Design review of the part built by this model. Coordinates are the model's own, in mm. Face numbers are marked on the shaded views. A direction names the side the tool comes from. Give positions to 0.01 mm unless a question says otherwise; leave off trailing zeros. Order: outer loops, then holes, each group sorted by start corner. A loop starts at its lowest first (then second) coordinate and runs counter-clockwise, first axis right, second up.
```python
from build123d import *

# Parameters (mm, degrees)
F0_W     = 149.768152
F0_H     = 37.856524
F1_DEPTH = 17
F2_W     = 12.044117
F2_H     = 10.517036
F3_DEPTH = 68.7
F2_W_2   = 49.102947
F2_H_2   = 8.573649
F4_DEPTH = 6.2


with BuildPart() as f1:
    # F0 (on Top) → F1 (new body)
    with BuildSketch(Plane.XY):
        with Locations((-0.134293, 0.313039)):
            Rectangle(F0_W, F0_H)
    extrude(amount=F1_DEPTH)

    # F2 (on face) → F3 (join)
    with BuildSketch(Plane.XY.offset(17)):
        with Locations((-0.08639, 13.982783)):
            Rectangle(F2_W, F2_H)
    extrude(amount=F3_DEPTH)

    # F2 (on face) → F4 (join)
    with BuildSketch(Plane.XY.offset(17)):
        with Locations((0.222437, -14.328398)):
            Rectangle(F2_W_2, F2_H_2)
    extrude(amount=F4_DEPTH)


solid = f1.part
```
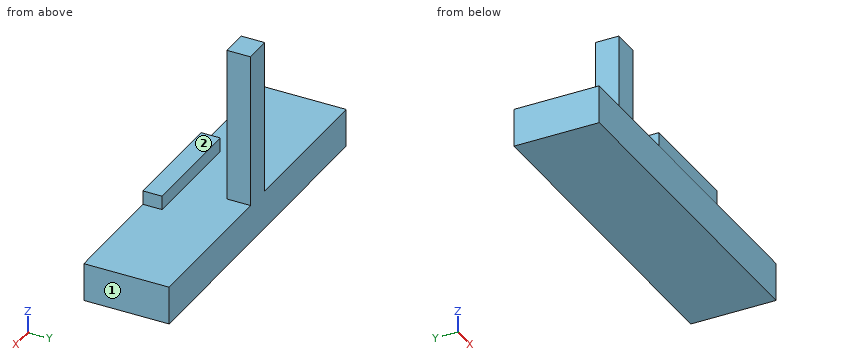
1. Take a section at D-D (y = -3.5). State the section outline as (x, z) points.
Recorded:
outline: (-75.02, 0) - (74.75, 0) - (74.75, 17) - (-75.02, 17) - close
2. Take a section at B-B (x = -2). State the section outline as (y, z) points.
Recorded:
outline: (-18.62, 0) - (19.24, 0) - (19.24, 85.7) - (8.72, 85.7) - (8.72, 17) - (-10.04, 17) - (-10.04, 23.2) - (-18.62, 23.2) - close
3. Take a section at C-C (z = 80). State the section outline as (x, y) points.
Recorded:
outline: (-6.11, 8.72) - (5.94, 8.72) - (5.94, 19.24) - (-6.11, 19.24) - close
4. For line 1 along Z through (x, y) = (-44.5, -5.5); line 2 along Y through (x, z) = (-2.5, 68.5); line 3 along X through (y, z) = (17, 71), list the stretches that pass through material, from the lowest coordinate up.
Recorded:
line 1: z = 0 to 17
line 2: y = 8.72 to 19.24
line 3: x = -6.11 to 5.94
5. Machinability: for the marked faces 1 and 2, which of the approach directions +Z, -Z, +X, -X, +Y, -Y give a long, thin tool a straight path to every point of the face, cutting with its end or side? Answer none if there is none.
Recorded:
face 1: +Z, -Z, +X, +Y, -Y
face 2: +Z, +X, -X, -Y
6. For pin 1 (1 mm diameter, centred on x = -13, y = -11.5, fed in from +Z); pin 2 (2 mm diameter, centred on x = -24, y = 3.5, fed in from +Z); pin 3 (6 mm diameter, centred on y = 9.5, z = 73, fed in from -X), all flat-tipped, find the tip position at first contact; note any pin that passes through.
Recorded:
pin 1: stops at z = 23.2
pin 2: stops at z = 17
pin 3: stops at x = -6.11
7. Take a section at A-A (y = 15.5). State the section outline as (x, z) points, then the cut area to 3 significant figures.
Recorded:
outline: (-75.02, 0) - (74.75, 0) - (74.75, 17) - (5.94, 17) - (5.94, 85.7) - (-6.11, 85.7) - (-6.11, 17) - (-75.02, 17) - close
area: 3,370 mm2
